```python
from build123d import *


with BuildPart() as part:
    # 草圖1 → 旋轉1 (revolve)
    with BuildSketch(Plane.XY):
        Polygon((4, -8), (4, 8), (15, 8), (15, 5.5), (18.62, 5.5), (18.62, -5.5), (15, -5.5), (15, -8), align=None)
    revolve(axis=Axis((0, 49.340027701, 0), (0, -1, 0)))

    # 草圖7 → 旋轉2 (revolve)
    with BuildSketch(Plane.XY):
        Polygon((-22.5, -6.5), (-18.62, -5.5), (-15, -5.5), (-15, -6.5), (-18.62, -6.5), (-22.5, -7.5), align=None)
    revolve_2 = revolve(axis=Axis((0, 0, 0), (0, 1, 0)))

    # 鏡射1: 旋轉2 across plane
    add(revolve_2.mirror(Plane.ZX))


solid = part.part
```
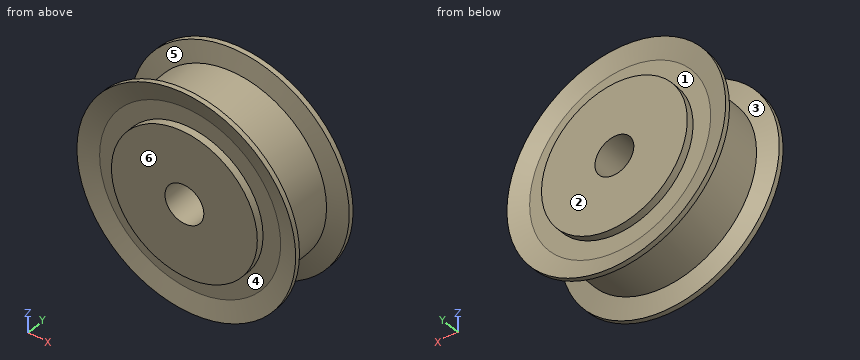
Part model, mm, in its own coordinate system. Face numbers are marked on the shaded views. A direction names the side the tool comes from. Round coordinates to 2 decimals unless told otherwise and drop trailing zeros. Order: outer loops, then holes, each group sorted by start corner. A loop starts at its lowest first (then second) coordinate and runs counter-clockwise, first axis right, second up. Notation, with made-up numbers: M 18.5,12.5 L 33.5,12.5 A10 ccw 33.5,26.5 Z; hole C 35,53 d11. An arc over 180 degrees is marked long. Put each result on its own line as item: value. Start each with the question number.
1. Tool access for the marked faces 1, 2 and 3: list every direction of +Z, -Z, +X, -X, +Y, -Y with a clear straight run to the whole face (end or side of a thin tool).
2. Slice it at A-A on z = 0. List the corners of the cut face in (x, y), then the cut area to 3 significant figures.
3. Drop flat-ended pins along their axis: pin 1 (6 mm diameter, centred on y = -6, z = -17, fed in from -X); pin 2 (8 mm diameter, centred on x = -13.5, z = 14, fed in from +Y); pin 3 (7 mm diameter, centred on x = 0, z = 0, fed in from +Y) (3 decimals); pin 4 (4 mm diameter, centred on y = 1, z = -10.5, fed in from -X). Give the stop position or say it passes through.
4. Slice it at C-C on y = 0.5. List the corners of the cut face in (x, z).
5. Two-plate mould, pull along X, no slides. Class the marked faces 4, 5 and 6: +X half, -X half, draft (parallel to the pull), parting line (faces both ways), or undercut.
6. Drill centre lines: probe 1 along Z at (x, y) = (0, -2.5); probe 2 along Y at (x, z) = (17.5, 1.5); probe 3 along Y at (x, z) = (16, -13). Where is each one in solid material? Low to high. Write a range as [from, to].
7. Slice it at B-B on x = 0. List the corners of the cut face in (y, z), then the cut area to 3 significant figures.
Findings:
1. face 1: +Y
1. face 2: +Z, -Z, +X, -X, +Y
1. face 3: none
2. outline: M -22.5,-7.5 L -18.62,-6.5 L -15,-6.5 L -15,-8 L -4,-8 L -4,8 L -15,8 L -15,6.5 L -18.62,6.5 L -22.5,7.5 L -22.5,6.5 L -18.62,5.5 L -18.62,-5.5 L -22.5,-6.5 Z; M 4,-8 L 15,-8 L 15,-6.5 L 18.62,-6.5 L 22.5,-7.5 L 22.5,-6.5 L 18.62,-5.5 L 18.62,5.5 L 22.5,6.5 L 22.5,7.5 L 18.62,6.5 L 15,6.5 L 15,8 L 4,8 Z
2. area: 462 mm2
3. pin 1: x = -17.58
3. pin 2: y = 7.5
3. pin 3: through
3. pin 4: x = -16.57
4. outline: C 0,0 d37.24; hole C 0,0 d8
5. face 4: undercut
5. face 5: parting line
5. face 6: draft
6. probe 1: [-18.62, -4], [4, 18.62]
6. probe 2: [-6.5, 6.5]
6. probe 3: [-7.01, -6.01], [6.01, 7.01]
7. outline: M -8,-15 L -6.5,-15 L -6.5,-18.62 L -7.5,-22.5 L -6.5,-22.5 L -5.5,-18.62 L 5.5,-18.62 L 6.5,-22.5 L 7.5,-22.5 L 6.5,-18.62 L 6.5,-15 L 8,-15 L 8,-4 L -8,-4 Z; M -8,4 L 8,4 L 8,15 L 6.5,15 L 6.5,18.62 L 7.5,22.5 L 6.5,22.5 L 5.5,18.62 L -5.5,18.62 L -6.5,22.5 L -7.5,22.5 L -6.5,18.62 L -6.5,15 L -8,15 Z
7. area: 462 mm2
